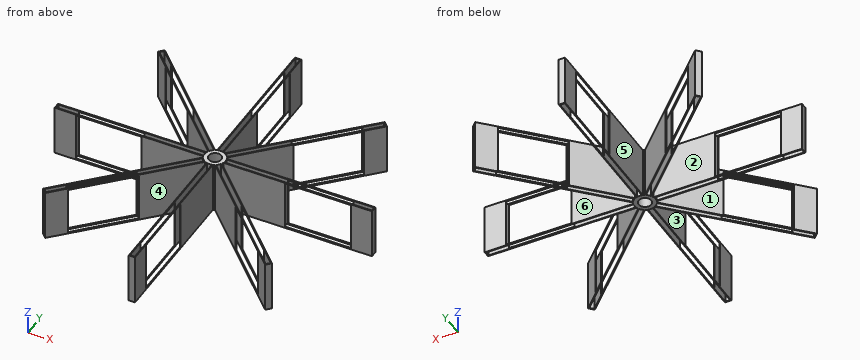
```python
from build123d import *

# Parameters (mm, degrees)
SKETCH1_R           = 25
BOSS_EXTRUDE1_DEPTH = 120
BOSS_EXTRUDE3_DEPTH = 120
SKETCH5_W           = 116
SKETCH5_H           = 155
CUT_EXTRUDE1_DEPTH  = 20
SKETCH6_W           = 116
SKETCH6_H           = 150
CUT_EXTRUDE2_DEPTH  = 20
SKETCH7_W           = 116
SKETCH7_H           = 155
CUT_EXTRUDE3_DEPTH  = 20
SKETCH8_W           = 155
SKETCH8_H           = 116
CUT_EXTRUDE4_DEPTH  = 20
SKETCH9_W           = 114
SKETCH9_H           = 155
CUT_EXTRUDE5_DEPTH  = 20
SKETCH10_W          = 155
SKETCH10_H          = 116
CUT_EXTRUDE6_DEPTH  = 20
SKETCH12_W          = 116
SKETCH12_H          = 155
CUT_EXTRUDE7_DEPTH  = 20
SKETCH13_W          = 116
SKETCH13_H          = 155
CUT_EXTRUDE8_DEPTH  = 20
SKETCH14_R          = 15
CUT_EXTRUDE11_DEPTH = 543.148846766


with BuildPart() as part:
    # Sketch1 → Boss-Extrude1 (new body)
    with BuildSketch(Plane.XY):
        Circle(SKETCH1_R)
    extrude(amount=BOSS_EXTRUDE1_DEPTH)

    # Sketch2 → Boss-Extrude3 (add)
    with BuildSketch(Plane.XY):
        with BuildLine():
            Line((11.560121095, 22.166722813), (259.04749451, 269.654096228))
            Line((259.04749451, 269.654096228), (269.654096228, 259.04749451))
            Line((269.654096228, 259.04749451), (22.166722813, 11.560121095))
            ThreePointArc((22.166722813, 11.560121095), (23.096988313, 9.567085809), (23.848480035, 7.5))
            Line((23.848480035, 7.5), (373.848480035, 7.5))
            Line((373.848480035, 7.5), (373.848480035, -7.5))
            Line((373.848480035, -7.5), (23.848480035, -7.5))
            ThreePointArc((23.848480035, -7.5), (23.096988313, -9.567085809), (22.166722813, -11.560121095))
            Line((22.166722813, -11.560121095), (269.654096228, -259.04749451))
            Line((269.654096228, -259.04749451), (259.04749451, -269.654096228))
            Line((259.04749451, -269.654096228), (11.560121095, -22.166722813))
            ThreePointArc((11.560121095, -22.166722813), (9.567085809, -23.096988313), (7.5, -23.848480035))
            Line((7.5, -23.848480035), (7.5, -373.848480035))
            Line((7.5, -373.848480035), (-7.5, -373.848480035))
            Line((-7.5, -373.848480035), (-7.5, -23.848480035))
            ThreePointArc((-7.5, -23.848480035), (-9.567085809, -23.096988313), (-11.560121095, -22.166722813))
            Line((-11.560121095, -22.166722813), (-259.04749451, -269.654096228))
            Line((-259.04749451, -269.654096228), (-269.654096228, -259.04749451))
            Line((-269.654096228, -259.04749451), (-22.166722813, -11.560121095))
            ThreePointArc((-22.166722813, -11.560121095), (-23.096988313, -9.567085809), (-23.848480035, -7.5))
            Line((-23.848480035, -7.5), (-373.848480035, -7.5))
            Line((-373.848480035, -7.5), (-373.848480035, 7.5))
            Line((-373.848480035, 7.5), (-23.848480035, 7.5))
            ThreePointArc((-23.848480035, 7.5), (-23.096988313, 9.567085809), (-22.166722813, 11.560121095))
            Line((-22.166722813, 11.560121095), (-269.654096228, 259.04749451))
            Line((-269.654096228, 259.04749451), (-259.04749451, 269.654096228))
            Line((-259.04749451, 269.654096228), (-11.560121095, 22.166722813))
            ThreePointArc((-11.560121095, 22.166722813), (-9.567085809, 23.096988313), (-7.5, 23.848480035))
            Line((-7.5, 23.848480035), (-7.5, 373.848480035))
            Line((-7.5, 373.848480035), (7.5, 373.848480035))
            Line((7.5, 373.848480035), (7.5, 23.848480035))
            ThreePointArc((7.5, 23.848480035), (9.567085809, 23.096988313), (11.560121095, 22.166722813))
        make_face()
        with BuildLine():
            Line((259.04749451, 266.825669103), (13.355477064, 21.133651658))
            ThreePointArc((13.355477064, 21.133651658), (17.67766953, 17.67766953), (21.133651658, 13.355477064))
            Line((21.133651658, 13.355477064), (266.825669103, 259.04749451))
            Line((266.825669103, 259.04749451), (259.04749451, 266.825669103))
        make_face(mode=Mode.SUBTRACT)
        with BuildLine():
            Line((-5.5, 371.848480035), (5.5, 371.848480035))
            Line((5.5, 371.848480035), (5.5, 24.387496797))
            ThreePointArc((5.5, 24.387496797), (0, 25), (-5.5, 24.387496797))
            Line((-5.5, 24.387496797), (-5.5, 371.848480035))
        make_face(mode=Mode.SUBTRACT)
        with BuildLine():
            Line((371.848480035, 5.5), (24.387496797, 5.5))
            ThreePointArc((24.387496797, 5.5), (25, 0), (24.387496797, -5.5))
            Line((24.387496797, -5.5), (371.848480035, -5.5))
            Line((371.848480035, -5.5), (371.848480035, 5.5))
        make_face(mode=Mode.SUBTRACT)
        with BuildLine():
            Line((266.825669103, -259.04749451), (21.133651658, -13.355477064))
            ThreePointArc((21.133651658, -13.355477064), (17.67766953, -17.67766953), (13.355477064, -21.133651658))
            Line((13.355477064, -21.133651658), (259.04749451, -266.825669103))
            Line((259.04749451, -266.825669103), (266.825669103, -259.04749451))
        make_face(mode=Mode.SUBTRACT)
        with BuildLine():
            Line((5.5, -371.848480035), (5.5, -24.387496797))
            ThreePointArc((5.5, -24.387496797), (0, -25), (-5.5, -24.387496797))
            Line((-5.5, -24.387496797), (-5.5, -371.848480035))
            Line((-5.5, -371.848480035), (5.5, -371.848480035))
        make_face(mode=Mode.SUBTRACT)
        with BuildLine():
            Line((-259.04749451, -266.825669103), (-13.355477064, -21.133651658))
            ThreePointArc((-13.355477064, -21.133651658), (-17.67766953, -17.67766953), (-21.133651658, -13.355477064))
            Line((-21.133651658, -13.355477064), (-266.825669103, -259.04749451))
            Line((-266.825669103, -259.04749451), (-259.04749451, -266.825669103))
        make_face(mode=Mode.SUBTRACT)
        with BuildLine():
            Line((-371.848480035, -5.5), (-24.387496797, -5.5))
            ThreePointArc((-24.387496797, -5.5), (-25, 0), (-24.387496797, 5.5))
            Line((-24.387496797, 5.5), (-371.848480035, 5.5))
            Line((-371.848480035, 5.5), (-371.848480035, -5.5))
        make_face(mode=Mode.SUBTRACT)
        with BuildLine():
            Line((-266.825669103, 259.04749451), (-21.133651658, 13.355477064))
            ThreePointArc((-21.133651658, 13.355477064), (-17.67766953, 17.67766953), (-13.355477064, 21.133651658))
            Line((-13.355477064, 21.133651658), (-259.04749451, 266.825669103))
            Line((-259.04749451, 266.825669103), (-266.825669103, 259.04749451))
        make_face(mode=Mode.SUBTRACT)
    extrude(amount=BOSS_EXTRUDE3_DEPTH)

    # Sketch5 → Cut-Extrude1 (cut)
    with BuildSketch(Plane(origin=(5.303300859, 5.303300859, 0), x_dir=(0, 0, -1), z_dir=(0.7071067811865304, 0.7071067811865648, 0))):
        with Locations((-60, 246.348480035)):
            Rectangle(SKETCH5_W, SKETCH5_H)
    extrude(amount=-CUT_EXTRUDE1_DEPTH, mode=Mode.SUBTRACT)

    # Sketch6 → Cut-Extrude2 (cut)
    with BuildSketch(Plane.ZY.offset(7.5)):
        with Locations((60, 248.848480035)):
            Rectangle(SKETCH6_W, SKETCH6_H)
    extrude(amount=-CUT_EXTRUDE2_DEPTH, mode=Mode.SUBTRACT)

    # Sketch7 → Cut-Extrude3 (cut)
    with BuildSketch(Plane(origin=(5.303300859, -5.303300859, 0), x_dir=(0, 0, -1), z_dir=(0.7071067811865477, -0.7071067811865475, 0))):
        with Locations((-60, 246.348480035)):
            Rectangle(SKETCH7_W, SKETCH7_H)
    extrude(amount=-CUT_EXTRUDE3_DEPTH, mode=Mode.SUBTRACT)

    # Sketch8 → Cut-Extrude4 (cut)
    with BuildSketch(Plane.XZ.offset(7.5)):
        with Locations((-246.348480035, 60)):
            Rectangle(SKETCH8_W, SKETCH8_H)
    extrude(amount=-CUT_EXTRUDE4_DEPTH, mode=Mode.SUBTRACT)

    # Sketch9 → Cut-Extrude5 (cut)
    with BuildSketch(Plane(origin=(-5.303300859, 5.303300859, 0), x_dir=(0, 0, 1), z_dir=(-0.7071067811865476, 0.7071067811865476, 0))):
        with Locations((59, -246.348480035)):
            Rectangle(SKETCH9_W, SKETCH9_H)
    extrude(amount=-CUT_EXTRUDE5_DEPTH, mode=Mode.SUBTRACT)

    # Sketch10 → Cut-Extrude6 (cut)
    with BuildSketch(Plane.XZ.offset(7.5)):
        with Locations((246.348480035, 60)):
            Rectangle(SKETCH10_W, SKETCH10_H)
    extrude(amount=-CUT_EXTRUDE6_DEPTH, mode=Mode.SUBTRACT)

    # Sketch12 → Cut-Extrude7 (cut)
    with BuildSketch(Plane.ZY.offset(7.5)):
        with Locations((60, -246.348480035)):
            Rectangle(SKETCH12_W, SKETCH12_H)
    extrude(amount=-CUT_EXTRUDE7_DEPTH, mode=Mode.SUBTRACT)

    # Sketch13 → Cut-Extrude8 (cut)
    with BuildSketch(Plane(origin=(-5.303300859, -5.303300859, 0), x_dir=(0, 0, 1), z_dir=(-0.7071067811865477, -0.7071067811865475, 0))):
        with Locations((60, -246.348480035)):
            Rectangle(SKETCH13_W, SKETCH13_H)
    extrude(amount=-CUT_EXTRUDE8_DEPTH, mode=Mode.SUBTRACT)

    # Sketch14 → Cut-Extrude11 (cut, through all)
    with BuildSketch(Plane(origin=(0, 0, 0), x_dir=(-1, 0, 0), z_dir=(0, 0, -1))):
        Circle(SKETCH14_R)
    extrude(amount=-CUT_EXTRUDE11_DEPTH, mode=Mode.SUBTRACT)


solid = part.part
```
The listing builds one solid part. Answer for the finished solid, in the listing's coordinates (mm). Face numbers are marked on the shaded views. A direction names the side the tool comes from. Give positions to 0.01 mm unless a question says otherwise; leave off trailing zeros. Write each loop counter-clockwise with the first axis right and the second up, starting at its lowest first coordinate (ties: lowest second). Pieces come first, ordered by that corner, then holes. Notation, with made-up numbers: (-7, -19) -> (20, -19) arc R23 cw to (20, -9) -> close; hole circle Ø11 at (-8.5, 56.5). An arc over 180 degrees is marked (long way). Write item = value, one per line. Start each with the question number.
1) The part is cut by section B-B, the plane z = 77.5. Count the separate pieces of the cut face and the enclosed holes in it, and give its area (3 significant figures).
2) Each of these flat-tipped pins is pushed along its axis until it touches: pin 1 (1.5 mm diameter, centred on x = 102, z = 47.5, fed in from +Y); pin 2 (8 mm diameter, centred on x = -115.5, z = 21, fed in from +Y); pin 3 (2 mm diameter, centred on x = 36, z = 50, fed in from +Y). Where does it stop, or does it pass through?
3) Which of the six approach directions +Z, -Z, +X, -X, +Y, -Y give full straight-line access (tool end or side, diameter ignored) to the marked faces 4, 5 and 6?
4) Determine the mould class of the marked faces 1, 2 and 3 for opening direction X: +X half, -X half, draft (parallel to the pull), parting line (faces both ways), or undercut.
5) The part is cut by section A-A, the plane y = 295.5. Determine the outline of the cut face in (x, z), and give its area (3 significant figures).
6) The part is cut by section C-C, the plane x = 35. Determine the outline of the cut face in (y, z).
7) Straight lines are drawn through the part: line 1 along Y through (x, z) = (0, 70.5); line 2 along X through (y, z) = (159, 96); line 3 along X through (y, z) = (117.5, 68.5). For each, find the intervals that lie inside material, in ascending order.
Solutions:
q1.separate_pieces = 9
q1.enclosed_holes = 1
q1.area = 7,680 mm²
q2.pin_1 = 113.36
q2.pin_2 = 124.7
q2.pin_3 = 47.61
q3.face_4 = +Z, -Z, -Y
q3.face_5 = +Z, -Z, +Y
q3.face_6 = +Z, -Z, +X
q4.face_1 = -X half
q4.face_2 = draft
q4.face_3 = undercut
q5.outline = (-7.5, 0) -> (-5.5, 0) -> (-5.5, 2) -> (-7.5, 2) -> close; (-7.5, 118) -> (-5.5, 118) -> (-5.5, 120) -> (-7.5, 120) -> close; (5.5, 0) -> (7.5, 0) -> (7.5, 2) -> (5.5, 2) -> close; (5.5, 118) -> (7.5, 118) -> (7.5, 120) -> (5.5, 120) -> close
q5.area = 16.0 mm²
q6.outline = (-45.61, 0) -> (-42.78, 0) -> (-42.78, 120) -> (-45.61, 120) -> close; (-27.22, 0) -> (-24.39, 0) -> (-24.39, 120) -> (-27.22, 120) -> close; (-7.5, 0) -> (-5.5, 0) -> (-5.5, 120) -> (-7.5, 120) -> close; (5.5, 0) -> (7.5, 0) -> (7.5, 120) -> (5.5, 120) -> close; (24.39, 0) -> (27.22, 0) -> (27.22, 120) -> (24.39, 120) -> close; (42.78, 0) -> (45.61, 0) -> (45.61, 120) -> (42.78, 120) -> close
q7.line_1 = -373.85 to -371.85, -25 to -15, 15 to 25, 371.85 to 373.85
q7.line_2 = -7.5 to -5.5, 5.5 to 7.5
q7.line_3 = -109.72 to -106.89, -7.5 to -5.5, 5.5 to 7.5, 106.89 to 109.72
